Check sheet for the modelled part. Datum: model origin and axes. Units: mm. A direction names the side the tool comes from. Coordinates: 2 decimals unless noted, no trailing zeros. Order: outer loops, then holes, each group sorted by start corner. A loop starts at its lowest first (then second) coordinate and runs counter-clockwise, first axis right, second up.
1. Draft check along X on faces 3 (the flat face through (-0.2, 8.2, 5)), 4 (the cylindrical face through (11.923, 3.755, 2.465)), 5 (the cylindrical face through (0.217, -3.226, 2.492)). Enter one of: released by +X, released by -X, zero draft, split by the parting line, or undercut.
2. Gauge pin test, flat ends, axial feed: pin 1 Ø8 at (x, y) = (-3, 10) entering from -Z; pin 2 Ø2.5 at (x, y) = (0, 2.25) entering from +Z; pin 3 Ø3 at (y, z) = (0, 10) entering from -X; pin 4 Ø3 at (x, z) = (2.5, 9) entering from -Y. Record the tip position at first contact, or that the pin passes through.
3. Cross-section at D-D (y = -7.25). Enter the section's corners in (x, z).
4. Thickness scan on line 1 (Y direction, x = 0, z = 1.6); line 2 (Z direction, x = -7.3, y = 0); line 3 (Y direction, x = 0.5, z = 4.25). Record the ranges inside material, lowest first.
5. Cross-section at B-B (y = 6.75). Enter the section's corners in (x, z), then the cut area to 3 significant figures.
6. Set-up check for faces 1 (the cylindrical face through (5.323, -2.769, 8.697)), 2 (the cylindrical face through (3.04, -0.61, 2.49)): record each of +Z, -Z, +X, -X, +Y, -Y from which the full face is reachable in a straight line by a thin tool's end or side.
7. Cross-section at A-A (z = 2.75). Enter the section's corners in (x, y), then the cut area to 3 significant figures.
8. Cross-section at C-C (z = 10.5). Enter the section's corners in (x, y), then the cut area to 3 significant figures.
```python
from build123d import *

# Parameters (mm, degrees)
SKIZZE1_R                            = 12.5
AUFSATZ_LINEAR_AUSTRAGEN1_DEPTH      = 40
SCHNITT_LINEAR_START                 = 30
SKIZZE4_R                            = 15
SKIZZE4_R_2                          = 12
SCHNITT_LINEAR_AUSTRAGEN1_DEPTH      = 20
SKIZZE5_R                            = 1.1
SCHNITT_LINEAR_AUSTRAGEN2_DEPTH      = 20
SKIZZE6_R                            = 1
SCHNITT_LINEAR_AUSTRAGEN3_DEPTH      = 10
SCHNITT_LINEAR_START_2               = 12.5
SKIZZE8_W                            = 25
SKIZZE8_H                            = 25
SCHNITT_LINEAR_AUSTRAGEN4_DEPTH      = 28.5
SKIZZE9_R                            = 1
SCHNITT_LINEAR_AUSTRAGEN5_DEPTH      = 13.5
SCHNITT_LINEAR_AUSTRAGEN5_DEPTH_BACK = 13.5
SKIZZE10_R                           = 1
SCHNITT_LINEAR_AUSTRAGEN6_DEPTH      = 13.5
SCHNITT_LINEAR_AUSTRAGEN6_DEPTH_BACK = 13.5


with BuildPart() as part:
    # Skizze1 → Aufsatz-Linear austragen1 (new body)
    with BuildSketch(Plane.XY):
        Circle(SKIZZE1_R)
    extrude(amount=AUFSATZ_LINEAR_AUSTRAGEN1_DEPTH)

    # Skizze2 → Schnitt-Rotation3 (revolve, cut)
    with BuildSketch(Plane(origin=(0, 0, 0), x_dir=(0, 0, -1), z_dir=(1, 0, 0))):
        Polygon((-35, -12.5), (-35, -8), (-5, -8), (-5, -12.5), (-33.974333956, -17.5), align=None)
    revolve(axis=Axis((0, 0, 40), (0, 0, -1)), mode=Mode.SUBTRACT)

    # Skizze4 → Schnitt-Linear austragen1 (cut)
    with BuildSketch(Plane.XY.offset(SCHNITT_LINEAR_START)):
        Circle(SKIZZE4_R)
        Circle(SKIZZE4_R_2, mode=Mode.SUBTRACT)
    extrude(amount=SCHNITT_LINEAR_AUSTRAGEN1_DEPTH, mode=Mode.SUBTRACT)

    # Skizze5 → Schnitt-Linear austragen2 (cut)
    with BuildSketch(Plane.XY.offset(40)):
        with Locations((-5.457266806, 6.503717322)):
            Circle(SKIZZE5_R)
        with Locations((6.503717322, 5.457266806)):
            Circle(SKIZZE5_R)
        with Locations((5.457266806, -6.503717322)):
            Circle(SKIZZE5_R)
        with Locations((-6.503717322, -5.457266806)):
            Circle(SKIZZE5_R)
    extrude(amount=-SCHNITT_LINEAR_AUSTRAGEN2_DEPTH, mode=Mode.SUBTRACT)

    # Skizze6 → Schnitt-Linear austragen3 (cut)
    with BuildSketch(Plane(origin=(0, 0, 0), x_dir=(-1, 0, 0), z_dir=(0, 0, -1))):
        with Locations((-2.25, 0)):
            Circle(SKIZZE6_R)
        with Locations((0, 2.25)):
            Circle(SKIZZE6_R)
        with Locations((2.25, 0)):
            Circle(SKIZZE6_R)
        with Locations((0, -2.25)):
            Circle(SKIZZE6_R)
    extrude(amount=-SCHNITT_LINEAR_AUSTRAGEN3_DEPTH, mode=Mode.SUBTRACT)

    # Skizze7 → Schnitt-Rotation4 (revolve, cut)
    with BuildSketch(Plane(origin=(0, 0, 0), x_dir=(0, 0, -1), z_dir=(1, 0, 0))):
        Polygon((-5.069914244, 0), (-35.074978214, 0), (-40, 0), (-42.313201415, 0), (-42.313201415, -6), (-40, -6), (-35, -6), (-5, -6), align=None)
    revolve(axis=Axis((0, 0, 40), (0, 0, -1)), mode=Mode.SUBTRACT)

    # Skizze8 → Schnitt-Linear austragen4 (cut, through all)
    with BuildSketch(Plane.XY.offset(SCHNITT_LINEAR_START_2)):
        Rectangle(SKIZZE8_W, SKIZZE8_H)
    extrude(amount=SCHNITT_LINEAR_AUSTRAGEN4_DEPTH, mode=Mode.SUBTRACT)

    # Skizze9 → Schnitt-Linear austragen5 (cut, two sides)
    with BuildSketch(Plane(origin=(0, 0, 0), x_dir=(0, 0, -1), z_dir=(1, 0, 0))) as schnitt_linear_austragen5_sk:
        with Locations((-10, 0)):
            Circle(SKIZZE9_R)
    extrude(amount=SCHNITT_LINEAR_AUSTRAGEN5_DEPTH, mode=Mode.SUBTRACT)
    extrude(schnitt_linear_austragen5_sk.sketch, amount=-SCHNITT_LINEAR_AUSTRAGEN5_DEPTH_BACK, mode=Mode.SUBTRACT)

    # Skizze10 → Schnitt-Linear austragen6 (cut, two sides)
    with BuildSketch(Plane(origin=(0, 0, 0), x_dir=(1, 0, 0), z_dir=(0, 1, 0))) as schnitt_linear_austragen6_sk:
        with Locations((0, -10)):
            Circle(SKIZZE10_R)
    extrude(amount=SCHNITT_LINEAR_AUSTRAGEN6_DEPTH, mode=Mode.SUBTRACT)
    extrude(schnitt_linear_austragen6_sk.sketch, amount=-SCHNITT_LINEAR_AUSTRAGEN6_DEPTH_BACK, mode=Mode.SUBTRACT)


solid = part.part
```
Data:
1. face 3: zero draft
1. face 4: split by the parting line
1. face 5: undercut
2. pin 1: stops at z = 0
2. pin 2: stops at z = 5.06
2. pin 3: stops at x = -8
2. pin 4: stops at y = -7.94
3. outline: (-10.18, 0) - (10.18, 0) - (10.18, 5) - (3.38, 5) - (3.38, 12.5) - (-3.38, 12.5) - (-3.38, 5) - (-10.18, 5) - close; hole circle Ø2 at (0, 10)
4. line 1: y = -12.5 to -3.25, -1.25 to 1.25, 3.25 to 12.5
4. line 2: z = 0 to 9, 11 to 12.5
4. line 3: y = -12.49 to -3.12, -1.38 to 1.38, 3.12 to 12.49
5. outline: (-10.52, 0) - (10.52, 0) - (10.52, 5) - (4.29, 5) - (4.29, 12.5) - (-4.29, 12.5) - (-4.29, 5) - (-10.52, 5) - close; hole circle Ø2 at (0, 10)
5. area: 166 mm2
6. face 1: +Z
6. face 2: +Z, -Z
7. outline: circle Ø25 at (0, 0); hole circle Ø2 at (-2.25, 0); hole circle Ø2 at (0, -2.25); hole circle Ø2 at (0, 2.25); hole circle Ø2 at (2.25, 0)
7. area: 478 mm2
8. outline: (-7.95, -0.87) arc R8 ccw to (-0.87, -7.95) - (-0.87, -5.94) arc R6 cw to (-5.94, -0.87) - close; (-7.95, 0.87) - (-5.94, 0.87) arc R6 cw to (-0.87, 5.94) - (-0.87, 7.95) arc R8 ccw to start; (0.87, -7.95) arc R8 ccw to (7.95, -0.87) - (5.94, -0.87) arc R6 cw to (0.87, -5.94) - close; (0.87, 5.94) arc R6 cw to (5.94, 0.87) - (7.95, 0.87) arc R8 ccw to (0.87, 7.95) - close
8. area: 74.1 mm2
